Build history of the part. All positions in model axes, mm. Face numbers are marked on the shaded views. Round coordinates to 2 decimals unless told otherwise and drop trailing zeros. Write each loop counter-clockwise with the first axis right and the second up, starting at its lowest first coordinate (ties: lowest second). Pieces come first, ordered by that corner, then holes. Notation, with made-up numbers: (7, 61) - (37, 61) arc R30 ccw to (37, 93) - close; hole circle Ø4 at (-6, 63). An arc over 180 degrees is marked (long way). Answer as a JSON object with one key per item and string values. Group by question number.
Item 1: Slice it at C-C, the plane y = 127.5. List the corners of the cut face in (x, z).
Item 2: Slice it at D-D, the plane x = 16.25. Give the number of separate pieces and of enclosed holes in the cut face, then the cut area to 3 significant figures.
Item 3: Flat gauge pins, fed straight in: pin 1 (2 mm diameter, centred on x = 20.5, y = 72, fed in from +Z); pin 2 (10 mm diameter, centred on x = 14, y = 26, fed in from +Z); pin 3 (5 mm diameter, centred on x = 16, y = 39.5, fed in from +Z); pin 4 (11 mm diameter, centred on y = -90.16, z = -90.16, fed in from +X). Where does each tip first touch, or does it go through?
Item 4: Slice it at A-A, the plane z = 0. List the corners of the cut face in (x, y).
Item 5: Probe line 1 (Z direction, x = 10, y = 0); line 2 (X direction, y = 130.5, z = 46.5); line 3 (Z direction, x = 1.75, y = 49.5). List the from-to ranges inside material, lowest first. Write a range as from..to.
Item 6: Two-plate mould, pull along Y, no slides. Class the marked faces 1, 2 and 3: +Y half, -Y half, draft (parallel to the pull), parting line (faces both ways), or undercut.
from build123d import *

# Parameters (mm, degrees)
F3_D     = 8.5
F3_DEPTH = 49.5
F3_TIP   = 2.5536576309


with BuildPart() as f1:
    # F0 (on Front) → F1 (revolve)
    with BuildSketch(Plane.XZ):
        Polygon((5.5, 115), (0, 115), (0, 107.5), (0, 103), (3, 103), (3, 107.5), (25, 107.5), (25, 142.5), (5.5, 142.5), align=None)
    revolve(axis=Axis((120.2051416039, 0, 0), (1, 0, 0)))

    # F3
    with Locations(Plane.YZ.offset(25)):
        with Locations((0, 127.5), (90.1561146013, 90.1561146013), (127.5, 0), (90.1561146013, -90.1561146013), (0, -127.5), (-90.1561146013, -90.1561146013), (-127.5, 0), (-90.1561146013, 90.1561146013)):
            Hole(F3_D / 2, depth=F3_DEPTH)
            with Locations((0, 0, -(F3_DEPTH + F3_TIP / 2))):  # 118° drill point
                Cone(0, F3_D / 2, F3_TIP, mode=Mode.SUBTRACT)


solid = f1.part
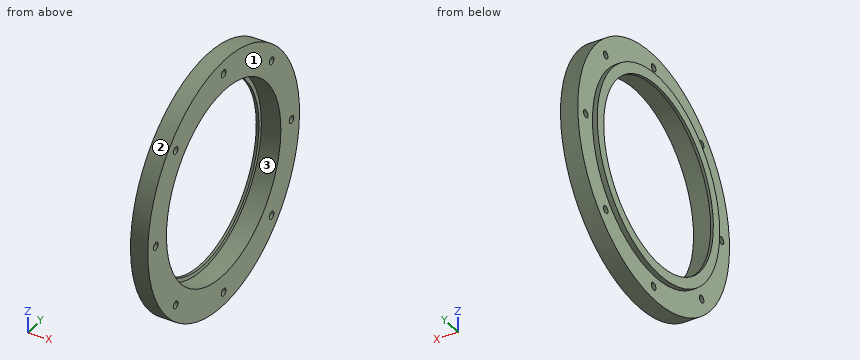
Geometry says:
{
 "1": {"outline": "(5.5, -63.64) - (25, -63.64) - (25, -4.25) - (5.5, -4.25) - close; (5.5, 4.25) - (25, 4.25) - (25, 63.64) - (5.5, 63.64) - close"},
 "2": {"separate pieces": "1", "enclosed holes": "9", "area": "27,000 mm^2"},
 "3": {"pin 1": "stops at z = 123.55", "pin 2": "stops at z = 140.94", "pin 3": "stops at z = 137.61", "pin 4": "stops at x = 25"},
 "4": {"outline": "(0, -115) - (5.5, -115) - (5.5, -123.25) - (25, -123.25) - (25, -107.5) - (3, -107.5) - (3, -103) - (0, -103) - close; (0, 103) - (3, 103) - (3, 107.5) - (25, 107.5) - (25, 123.25) - (5.5, 123.25) - (5.5, 115) - (0, 115) - close; (5.5, -142.5) - (25, -142.5) - (25, -131.75) - (5.5, -131.75) - close; (5.5, 131.75) - (25, 131.75) - (25, 142.5) - (5.5, 142.5) - close"},
 "5": {"line 1": "z = -142.5..-131.75, -123.25..-107.5, 107.5..123.25, 131.75..142.5", "line 2": "x = 5.5..25", "line 3": "z = -103.8..-90.33, 90.33..103.8"},
 "6": {"face 1": "draft", "face 2": "parting line", "face 3": "undercut"}
}
